Source: CAD feature listing. Evaluate the final solid. Frame: model axes, mm. Face numbers are marked on the shaded views. A direction names the side the tool comes from. Give positions to 0.01 mm unless a question says otherwise; leave off trailing zeros. Loops run counter-clockwise (first coordinate to the right, second up) from the corner with the lowest first, then second, coordinate; pieces in that order, holes last.
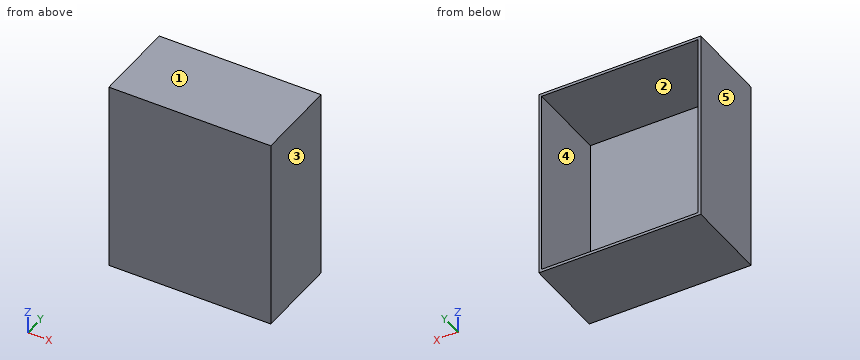
from build123d import *

# Parameters (mm, degrees)
F0_W     = 255.4635107517
F0_H     = 167.3530042171
F1_DEPTH = 127
F3_W     = 146.4032530785
F3_H     = 174.0650087595
F4_DEPTH = 76.2
F5_T     = -2.54


with BuildPart() as f1:
    # F0 (on Front) → F1 (new body)
    with BuildSketch(Plane.XZ):
        Rectangle(F0_W, F0_H)
    extrude(amount=F1_DEPTH)


with BuildPart() as f4:
    # F3 (on Front) → F4 (new body)
    with BuildSketch(Plane.XZ):
        Rectangle(F3_W, F3_H)
    extrude(amount=F4_DEPTH)

    # F5
    f5_openings = [f4.faces().sort_by_distance(p)[0] for p in [
        (0, 0, 0),
    ]]
    offset(amount=F5_T, openings=f5_openings)


solid = f4.part
1) Cut plane B-B (x = -12). Return loops of the section in (y, z).
Checks:
outline: (-76.2, -87.03) - (0, -87.03) - (0, -84.49) - (-73.66, -84.49) - (-73.66, 84.49) - (0, 84.49) - (0, 87.03) - (-76.2, 87.03) - close
2) Contact query for a flat-ended pin moving along its axis: P1, Ø10, axis at x = -55.5, z = -45.5, coming from the +Y side. Output: stop coordinate, or through.
Checks:
P1: stops at y = -73.66
3) Cut plane C-C (z = 44). Return loops of the section in (x, y).
Checks:
outline: (-73.2, -76.2) - (73.2, -76.2) - (73.2, 0) - (70.66, 0) - (70.66, -73.66) - (-70.66, -73.66) - (-70.66, 0) - (-73.2, 0) - close
4) Ray query, probe 1 along X at (y, z) = (-20.5, 58.5); probe 2 along Z at (x, y) = (-42, -66.5); probe 3 along Y at (x, z) = (-64.5, -32). Return the intervals inside material, ascending.
Checks:
probe 1: x = -73.2 to -70.66, 70.66 to 73.2
probe 2: z = -87.03 to -84.49, 84.49 to 87.03
probe 3: y = -76.2 to -73.66
5) Reachability of the marked faces 4 and 5 from +Z, -Z, +X, -X, +Y, -Y: full face, straight path, thin tool, end or side. Return the list, or none.
Checks:
face 4: +Y
face 5: +Z, -Z, -X, +Y, -Y
6) Pull-direction query (Z, two-part tool) for the marked faces 1, 2 and 3; classes: released by +Z, released by -Z, zero draft, split by the parting line, or undercut.
Checks:
face 1: released by +Z
face 2: undercut
face 3: zero draft
7) Cut plane A-A (y = -12). Return loops of the section in (x, z), and give its area (3 significant figures).
Checks:
outline: (-73.2, -87.03) - (73.2, -87.03) - (73.2, 87.03) - (-73.2, 87.03) - close; hole (-70.66, -84.49) - (70.66, -84.49) - (70.66, 84.49) - (-70.66, 84.49) - close
area: 1,600 mm2
